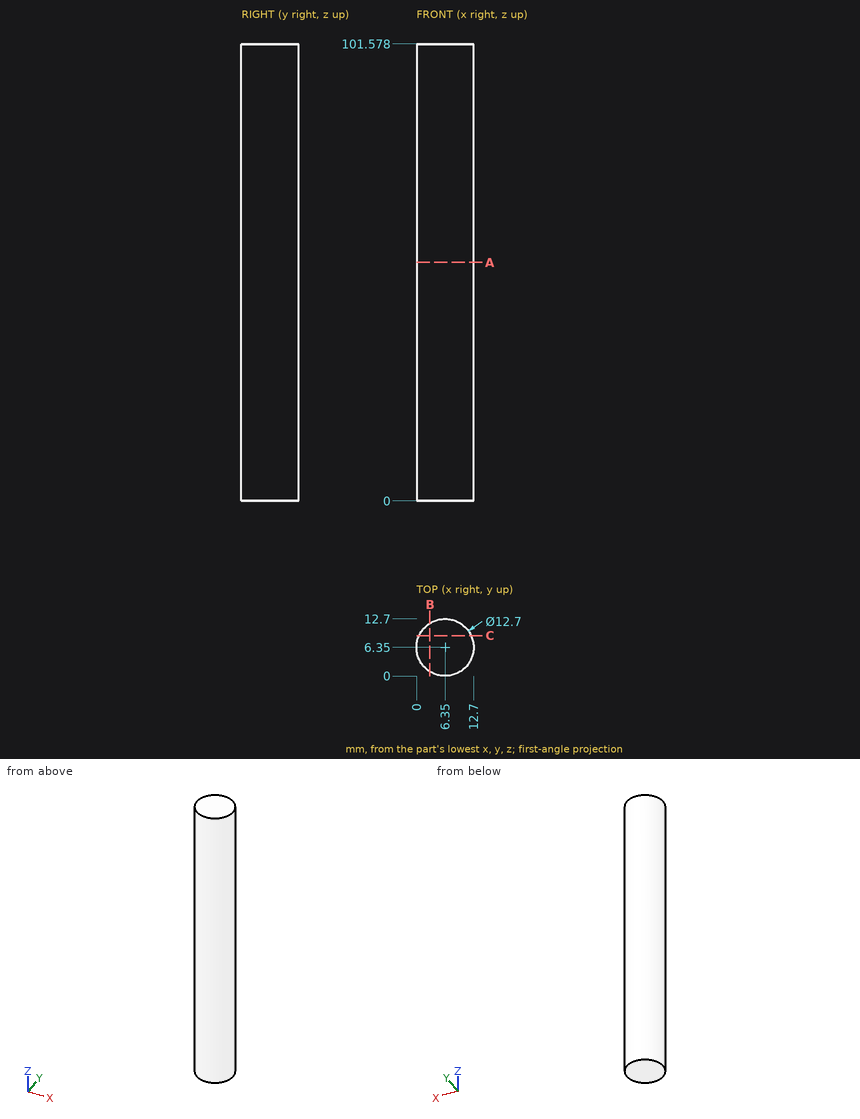
Verification items for this drawing (mm, ordinates from the low corner). Coordinates: 2 decimals unless noted, no trailing zeros. Write each loop counter-clockwise with the first axis right and the second up, starting at its lowest first coordinate (ties: lowest second). Pieces come first, ordered by that corner, then holes. Notation, with made-up numbers: M 2,21 L 44,21 A28 ccw 44,51 Z; hole C 54,27.25 d11. An arc over 180 degrees is marked long. Use one line per item in the form item = value. Start each with the question number.
1) Thickness scan on probe 1 along X at (y, z) = (6, 41.5); probe 2 along Y at (x, z) = (11.75, 77). Record the ranges inside material, lowest first. Write a range as from..to.
2) Go/stop test with flat-tipped pins: pin 1 Ø4 at (x, z) = (8.5, 32) entering from -Y; pin 2 Ø2 at (x, z) = (8.5, 38) entering from -Y (1 decimal); pin 3 Ø3 at (x, z) = (4.5, 86) entering from +Y. Record where each tip stops, or that it passes through.
3) Section check B-B on x = 3. Enter the section's corners in (y, z) (1 decimal), and give its area (3 significant figures).
4) Section check C-C on y = 9. Enter the section's corners in (x, z).
5) Section check A-A on z = 53. Enter the section's corners in (x, y).
Responses:
q1.probe_1 = 0.01..12.69
q1.probe_2 = 3.01..9.69
q2.pin_1 = 0
q2.pin_2 = 0.1
q2.pin_3 = 12.69
q3.outline = M 1,0 L 11.7,0 L 11.7,101.6 L 1,101.6 Z
q3.area = 1,100 mm2
q4.outline = M 0.58,0 L 12.12,0 L 12.12,101.58 L 0.58,101.58 Z
q5.outline = C 6.35,6.35 d12.7
